Autodesk Inventor part; units mm, degrees
ref_plane "YZ Plane" through (0, 0, 0) normal (1, 0, 0) x (0, 1, 0)
ref_plane "XZ Plane" through (0, 0, 0) normal (0, 1, 0) x (-1, 0, 0)
ref_plane "XY Plane" through (0, 0, 0) normal (0, 0, 1) x (1, 0, 0)
sketch "Sketch1" plane through (0, 0, 0) normal (0, 0, 1) x (1, 0, 0)
  line L0 (15.7385, -0.0311) -> (-29.1749, -0.0311)
  line L1 (-29.1749, -0.0311) -> (2.0558, -0.0311) construction
  line L2 (-29.1749, -8.0311) -> (-19.1749, -8.0311)
  line L3 (-19.1749, -8.0311) -> (-9.0765, -8.6728) construction
  line L4 (-9.0765, -8.6728) -> (-1.6699, -24.4547) construction
  spline S0 degree 2 poles (-19.1749, -8.0311) (-9.0765, -8.6728) (-1.6699, -24.4547) knots 1 1 1 2 2 2
  line L5 (-1.6699, -24.4547) -> (2.9761, -22.4111) construction
  line L6 (2.9761, -22.4111) -> (-2.9231, -11.7108) construction
  spline S1 degree 2 poles (-1.6699, -24.4547) (2.9761, -22.4111) (-2.9231, -11.7108) knots 1 1 1 2 2 2
  line L7 (-2.9231, -11.7108) -> (-2.9231, -4.7242) construction
  line L8 (-2.9231, -4.7242) -> (18.0519, -6.1311) construction
  line L9 (18.0519, -6.1311) -> (15.7385, -0.0311) construction
  spline S2 degree 3 poles (-2.9231, -11.7108) (-2.9231, -4.7242) (18.0519, -6.1311) (15.7385, -0.0311) knots 1 1 1 1 2 2 2 2
  arc A0 (-29.1749, -0.0311) -> (-29.1749, -8.0311) centre (-29.1749, -4.0311) ccw
  circle A1 centre (-29.1749, -4.0311) radius 2.15
  point P0 (0, 0)
  dimension "d0" = 8
  dimension "d1" = 10
  dimension "d2" = 4.3
extrude "Extrusion1" add sketch "Sketch1" along normal blind 3
sketch "Sketch2" plane through (0, 0, 3) normal (0, 0, 1) x (1, 0, 0)
  line L0 (15.7385, -0.0311) -> (-29.1749, -0.0311)
  line L1 (-29.1749, -0.0311) -> (-1.8249, -0.0311)
  circle A0 centre (-1.8249, -0.0311) radius 3.5
  point P0 (0, 0)
  dimension "d5" = 27.35
  dimension "d6" = 7
extrude "Extrusion2" cut sketch "Sketch2" against normal blind 3
sketch "Sketch3" plane through (0, 0, 3) normal (0, 0, 1) x (1, 0, 0)
  line L0 (-1.6699, -24.4547) -> (-2.4199, -23.1557)
  line L1 (-1.6699, -24.4547) -> (-0.1699, -24.4547) construction
  line L2 (-3.7341, -20.8795) -> (-2.4199, -23.1557)
  line L3 (-2.4199, -23.1557) -> (-1.13, -22.0176) construction
  line L4 (-1.13, -22.0176) -> (-2.0449, -20.2761) construction
  line L5 (-2.0449, -20.2761) -> (-3.7341, -20.8795) construction
  spline S0 degree 3 poles (-2.4199, -23.1557) (-1.13, -22.0176) (-2.0449, -20.2761) (-3.7341, -20.8795) knots 1 1 1 1 2 2 2 2
  point P0 (0, 0)
  dimension "d9" = 1.5
  dimension "d10" = 120
extrude "Extrusion3" cut sketch "Sketch3" against normal blind 3
fillet "Fillet2" radius 2 1 edges at (-3.5248, -20.8155, 1.5)
chamfer "Chamfer1" distance 1.2 angle 45 1 edges at (-31.3249, -4.0311, 0)
fillet "Fillet4" radius 1 2 edges at (1.6751, -0.0311, 1.5) (-5.3249, -0.0311, 1.5)
properties part number "retreat"
The listing builds one solid part. Answer for the finished solid, in the listing's coordinates (mm). A direction names the side the tool comes from. Coordinates: 2 decimals unless noted, no trailing zeros. Write each loop counter-clockwise with the first axis right and the second up, starting at its lowest first coordinate (ties: lowest second). Pieces come first, ordered by that corner, then holes. Notation, with made-up numbers: (50, -8.75) - (107, -8.75) arc R31 ccw to (107, 25.25) - close; hole circle Ø10 at (-9.5, -36). An arc over 180 degrees is marked (long way). Return JSON: item names as keys, results as strings. Group by question number.
Q1. Which of the six approach directions +Z, -Z, +X, -X, +Y, -Y give full straight-line access (tool end or side, diameter ignored) to faces 4 (the flat face through (-10, -6, 3)), 5 (the cylindrical face through (1.932, -0.255, 1.479))?
Q2. Find the intervals of material crossed by line 1 along X through (y, z) = (-3, 0.45); line 2 along X through (y, z) = (-1.75, 0.35); line 3 along Y through (x, z) = (-31, 2.8), in increasing order. Write a range as [from, to].
Q3. The part is cut by section A-A on x = -20. Write down the section's boundary in (y, z).
Q4. For a pull along X with two mould halves and no side action, classify faces 1 (the flat face through (-24, -8.031, 1)), 2 (the cylindrical face through (-5.581, -0.255, 1.521)), 3 (the cylindrical face through (-33.174, -4.119, 1.479)) as +X half, -X half, draft (parallel to the pull), parting line (faces both ways), or undercut.
Q5. A flat-ended cylindrical pin translates along its axis: pin 1 Ø8 at (x, y) = (1.5, -4.5) entering from -Z. Find the tip coordinate at first contact, or state that the pin passes through.
Evaluation:
{
 "1": {"face 4": "+Z, +X, -X, +Y, -Y", "face 5": "+Z, -Z, +Y"},
 "2": {"line 1": "x = [-33.04, -31.89], [-26.46, -3.68], [0.03, 14.57]", "line 2": "x = [-32.46, -31.12], [-27.23, -4.87], [1.22, 15.74]", "line 3": "y = [-7.59, -5.17], [-2.89, -0.47]"},
 "3": {"outline": "(-8.03, 0) - (-0.03, 0) - (-0.03, 3) - (-8.03, 3) - close"},
 "4": {"face 1": "draft", "face 2": "undercut", "face 3": "-X half"},
 "5": {"pin 1": "stops at z = 0"}
}
